Check sheet for the modelled part. Datum: model origin and axes. Units: mm. Face numbers are marked on the shaded views. A direction names the side the tool comes from. Coordinates: 2 decimals unless noted, no trailing zeros. Write each loop counter-clockwise with the first axis right and the second up, starting at its lowest first coordinate (ties: lowest second). Pieces come first, ordered by that corner, then holes. Notation, with made-up numbers: (49.5, -37.75) - (82.5, -37.75) arc R25 cw to (82.5, -22.75) - close; hole circle Ø5 at (27, 70). An arc over 180 degrees is marked (long way). Write each question's results on one line, items separated by ' | '.
from build123d import *

# Parameters (mm, degrees)
F1_DEPTH = 1.5875
F2_R     = 3.175
F3_DEPTH = 76.2
F4_COUNT = 8
F4_ANGLE = 315


with BuildPart() as f1:
    # F0 (on Front) → F1 (new body, symmetric)
    with BuildSketch(Plane.XZ):
        with BuildLine():
            Line((90.17, 6.35), (0, 6.35))
            Line((0, 6.35), (0, -6.35))
            Line((0, -6.35), (90.17, -6.35))
            ThreePointArc((90.17, -6.35), (150.4612042695, 0), (90.17, 6.35))
        make_face()
    extrude(amount=F1_DEPTH, both=True)

    # F2 (on Top) → F3 (join, symmetric)
    with BuildSketch(Plane.XY):
        Circle(F2_R)
    extrude(amount=F3_DEPTH, both=True)

    # F4: F1 ×8 about axis
    f4_axis = Axis((0, 0, 0), (0, 0, 1))


with BuildPart() as f1_1:
    add(f1.part)
    for i in range(1, F4_COUNT):
        add(f1.part.rotate(f4_axis, i * F4_ANGLE / (F4_COUNT - 1)))


solid = f1_1.part
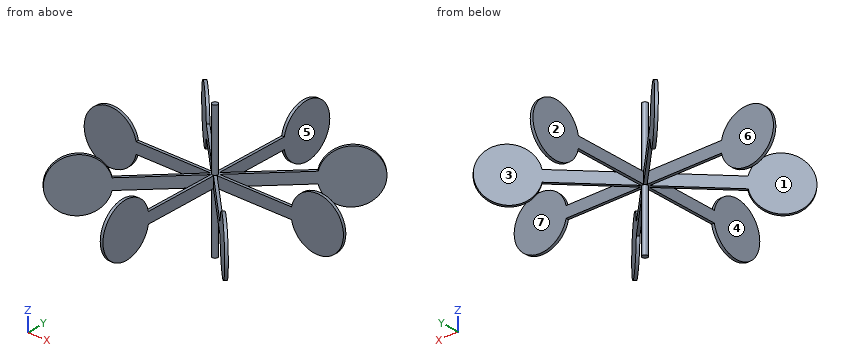
1. Sectioned sample at C-C (x = -117.5). Record the cut outline in (y, z).
Values follow:
outline: (-1.59, -30.38) - (1.59, -30.38) - (1.59, 30.38) - (-1.59, 30.38) - close
2. Material ranges on L1, parallel to X at y = 95, z = -17; L2, parallel to Y at x = -1.5, z = 12; L3, parallel to Y at x = -59, z = 1.5, recorded low to high. Write a range as [from, to].
Values follow:
L1: x = [-97.25, -92.75], [-1.59, 1.59], [92.75, 97.25] | L2: y = [-148, -91.96], [-2.8, 2.8], [91.96, 148] | L3: y = [-61.25, -56.75], [-1.59, 1.59], [56.75, 61.25]
3. Access from +Z, -Z, +X, -X, +Y, -Y to the whole of each face (thin tool, end or side, straight path). Record for the marked faces 4, 5, 6 and 7.
Values follow:
face 4: +Z, -Z, -Y | face 5: +Z, -Z, +Y | face 6: +Z, -Z, -X | face 7: +Z, -Z, +X
4. Sectioned sample at D-D (z = 47). Record the cut outline in (x, y) (3 decimals), then the cut area to 3 significant figures.
Values follow:
outline: circle Ø6.35 at (0, 0) | area: 31.7 mm^2
5. Sectioned sample at B-B (z = 0). Record the cut outline in (x, y).
Values follow:
outline: (-150.46, -1.59) - (-3.83, -1.59) - (-107.51, -105.27) - (-105.27, -107.51) - (-1.59, -3.83) - (-1.59, -150.46) - (1.59, -150.46) - (1.59, -3.83) - (105.27, -107.51) - (107.51, -105.27) - (3.83, -1.59) - (150.46, -1.59) - (150.46, 1.59) - (3.83, 1.59) - (107.51, 105.27) - (105.27, 107.51) - (1.59, 3.83) - (1.59, 150.46) - (-1.59, 150.46) - (-1.59, 3.83) - (-105.27, 107.51) - (-107.51, 105.27) - (-3.83, 1.59) - (-150.46, 1.59) - close
6. Sectioned sample at A-A (y = -8). Record the cut outline in (x, z), then the cut area to 3 significant figures.
Values follow:
outline: (-10.25, -6.35) - (-5.75, -6.35) - (-5.75, 6.35) - (-10.25, 6.35) - close; (-1.59, -6.35) - (1.59, -6.35) - (1.59, 6.35) - (-1.59, 6.35) - close; (5.75, -6.35) - (10.25, -6.35) - (10.25, 6.35) - (5.75, 6.35) - close | area: 154 mm^2
7. Go/stop test with flat-tipped pins: pin 1 (12 mm diameter, centred on x = -64, z = -13.5, fed in from +Y); pin 2 (18.5 mm diameter, centred on x = 64, z = -11.5, fed in from +Y); pin 3 (2 mm diameter, centred on x = -45.5, z = 1.5, fed in from +Y). Record where each tip stops, or that it passes through.
Values follow:
pin 1: stops at y = 72.25 | pin 2: stops at y = 75.5 | pin 3: stops at y = 48.75
8. Draft check along Y on the marked faces 1, 2 and 3. Enter one of: pulls with the +Y half, pulls with the -Y half, needs draft (parallel to the pull), parting line crosses it, or undercut.
Values follow:
face 1: undercut | face 2: needs draft | face 3: pulls with the +Y half
